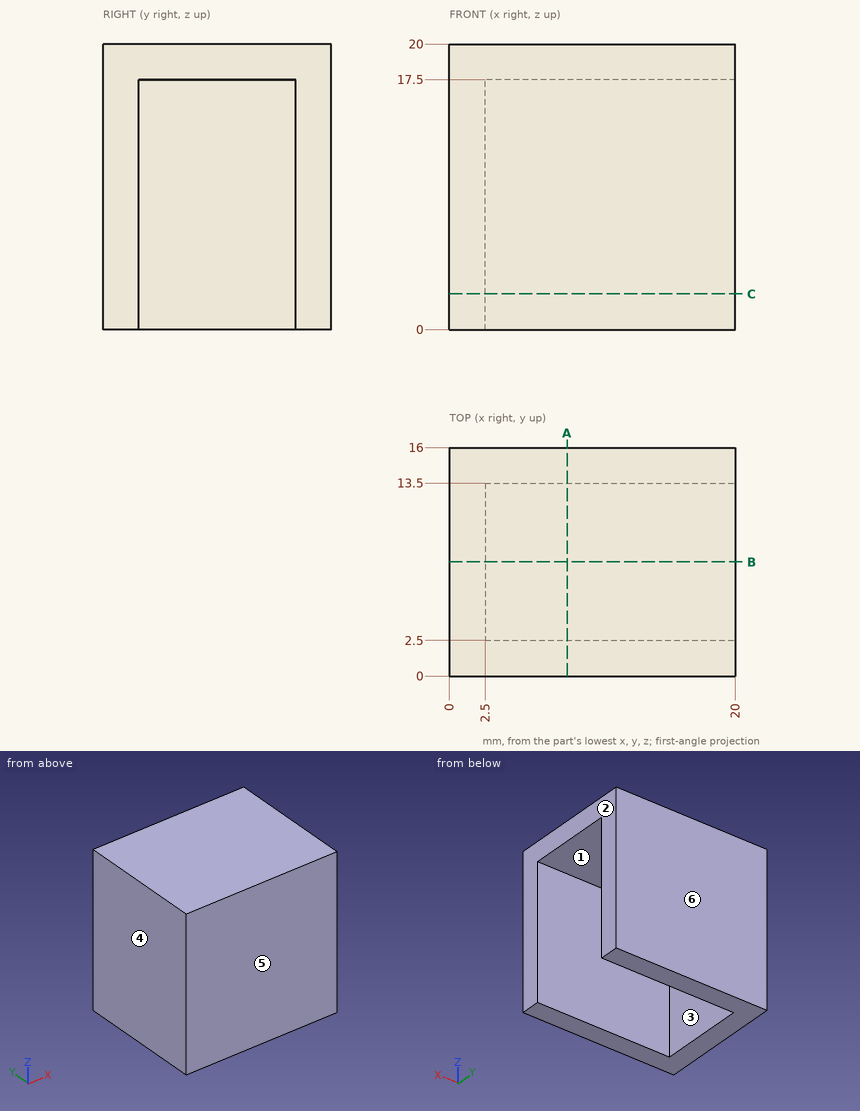
Here's the drawing with two shaded views (mm, measured from the low corner). I have some questions. A direction names the side the tool comes from. Give positions to 0.01 mm unless a question says otherwise; leave off trailing zeros. Loops run counter-clockwise (first coordinate to the right, second up) from the corner with the lowest first, then second, coordinate; pieces in that order, holes last. Notation, with made-up numbers: (-29, 61) - (18, 61) arc R6 cw to (18, 68) - close; hole circle Ø4 at (53, -2.75). An arc over 180 degrees is marked (long way). Answer in a Markdown table with one row per item. Add a question column.
Q1. For pin 1 (3.5 mm diameter, centred on y = 10.5, z = 13, fed in from +X); pin 2 (5.5 mm diameter, centred on x = 11.5, y = 8, fed in from -Z), each with a flat end and sliding along its axis, tell me the tip position at first contact or that it passes through.
Q2. Please list where these lines run through material, in increasing order: L1, parallel to Y at x = 16.5, z = 4.25; L2, parallel to X at y = 3, z = 14.75; L3, parallel to Z at x = 7, y = 9.5. Write a range as from..to.
Q3. If we section it at C-C (z = 2.5): List the corners of the cut face in (x, y) for me, plus the area to 4 significant figures.
Q4. If we section it at B-B (y = 8): List the corners of the cut face in (x, z) for me.
Q5. If we section it at A-A (x = 8.25): List the corners of the cut face in (y, z) for me.
Q6. We'd pull the mould along Y, two halves only. Please class the marked faces 3, 4, 5 and 6: +Y half, -Y half, draft (parallel to the pull), parting line (faces both ways), or undercut.
Q7. Which directions (+Z, -Z, +X, -X, +Y, -Y) give clear straight access to the entire face, cutting with the end or side of a thin tool? Please do the marked faces 1 and 2.
The answers:
| question | item | result |
|---|---|---|
| 1 | pin 1 | stops at x = 2.5 |
| 1 | pin 2 | stops at z = 17.5 |
| 2 | L1 | y = 0..2.5, 13.5..16 |
| 2 | L2 | x = 0..2.5 |
| 2 | L3 | z = 17.5..20 |
| 3 | outline | (0, 0) - (20, 0) - (20, 2.5) - (2.5, 2.5) - (2.5, 13.5) - (20, 13.5) - (20, 16) - (0, 16) - close |
| 3 | area | 127.5 mm^2 |
| 4 | outline | (0, 0) - (2.5, 0) - (2.5, 17.5) - (20, 17.5) - (20, 20) - (0, 20) - close |
| 5 | outline | (0, 0) - (2.5, 0) - (2.5, 17.5) - (13.5, 17.5) - (13.5, 0) - (16, 0) - (16, 20) - (0, 20) - close |
| 6 | face 3 | undercut |
| 6 | face 4 | draft |
| 6 | face 5 | -Y half |
| 6 | face 6 | +Y half |
| 7 | face 1 | -Z, +X |
| 7 | face 2 | +Z, -Z, +X, +Y, -Y |
